Geometry check sheet. Reference: the model listing, model coordinates, mm. A direction names the side the tool comes from. Round coordinates to 2 decimals unless told otherwise and drop trailing zeros. Write each loop counter-clockwise with the first axis right and the second up, starting at its lowest first coordinate (ties: lowest second). Pieces come first, ordered by that corner, then holes. Notation, with made-up numbers: M -36,82 L 9,82 A19 cw 9,118 Z; hole C 51.5,19.5 d5. An arc over 180 degrees is marked long. Answer as CSV lines item,"result". Start each with the question number.
```python
from build123d import *

# Parameters (mm, degrees)
F0_W     = 4.6228
F0_H     = 4.6228
F0_R     = 2.3114
F1_DEPTH = 3.175


with BuildPart() as f1:
    # F0 (on Front) → F1 (new body)
    with BuildSketch(Plane.XZ):
        with BuildLine():
            ThreePointArc((17.3114, -8.3125), (15, -6.0011), (12.6886, -8.3125))
            ThreePointArc((12.6886, -8.3125), (15, -10.6239), (17.3114, -8.3125))
        make_face()
        Polygon((100, -26.9875), (100, 26.9875), (80, 26.9875), (80, 30.1625), (0, 30.1625), (0, -8.3125), (0, -26.9875), align=None)
        with Locations((65.075, -16.3125)):
            Rectangle(F0_W, F0_H, mode=Mode.SUBTRACT)
        with BuildLine():
            ThreePointArc((17.3114, -8.3125), (15, -10.6239), (12.6886, -8.3125))
            ThreePointArc((12.6886, -8.3125), (15, -6.0011), (17.3114, -8.3125))
        make_face(mode=Mode.SUBTRACT)
        with Locations((65.075, -3.6125)):
            Rectangle(F0_W, F0_H, mode=Mode.SUBTRACT)
        with Locations((65.075, 9.0875)):
            Rectangle(F0_W, F0_H, mode=Mode.SUBTRACT)
        Polygon((-65.075, -26.9875), (0, -26.9875), (0, -8.3125), (0, 30.1625), (-80, 30.1625), (-80, 26.9875), (-100, 26.9875), (-100, -26.9875), align=None)
        with Locations((-65.075, -16.3125)):
            Rectangle(F0_W, F0_H, mode=Mode.SUBTRACT)
        with Locations((-65.075, -3.6125)):
            Rectangle(F0_W, F0_H, mode=Mode.SUBTRACT)
        with Locations((-15, -8.3125)):
            Circle(F0_R, mode=Mode.SUBTRACT)
        with Locations((-65.075, 9.0875)):
            Rectangle(F0_W, F0_H, mode=Mode.SUBTRACT)
    extrude(amount=F1_DEPTH)


solid = f1.part
```
1) Section check A-A, the plane x = -15. Record the cut outline in (y, z) (1 decimal), plus the area to 3 significant figures.
2) Scan lines: line 1 (X direction, y = -2.4, z = -4); line 2 (Z direction, x = -15, y = -1.15); line 3 (Z direction, x = 64.5, y = -1.1). Record each from-to range of solid material in increasing order. Write a range as from..to.
3) Section check C-C, the plane y = -1.85. Give the number of separate pieces and of enclosed holes in the cut face, plus the area to 3 significant figures.
4) Access from +Z, -Z, +X, -X, +Y, -Y to the whole of each face (thin tool, end or side, straight path). Record for faces 4 (the flat face through (1, -2, 30.162)), 5 (the flat face through (65, -2, 11.399)).
5) Section check B-B, the plane z = 8.5. Record the cut outline in (x, y) (3 decimals).
6) Mould release check, pull along Z, two halves, no side actions. Record for faces 1 (the flat face through (100, -2, 0)), 2 (the flat face through (-67.386, -2, 9)), 3 (the flat face through (90, -2, 26.988)): released by +Z, released by -Z, zero draft, split by the parting line, or undercut.
Results:
1,outline,"M -3.2,-27 L 0,-27 L 0,-10.6 L -3.2,-10.6 Z; M -3.2,-6 L 0,-6 L 0,30.2 L -3.2,30.2 Z"
1,area,"167 mm^2"
2,line 1,"x = -100..-67.39, -62.76..62.76, 67.39..100"
2,line 2,"z = -26.99..-10.62, -6..30.16"
2,line 3,"z = -26.99..-18.62, -14..-5.92, -1.3..6.78, 11.4..30.16"
3,separate pieces,"1"
3,enclosed holes,"8"
3,area,"11,100 mm^2"
4,face 4,"+Z, +X, -X, +Y, -Y"
4,face 5,"+Y, -Y"
5,outline,"M -100,-3.175 L -67.386,-3.175 L -67.386,0 L -100,0 Z; M -62.764,-3.175 L 62.764,-3.175 L 62.764,0 L -62.764,0 Z; M 67.386,-3.175 L 100,-3.175 L 100,0 L 67.386,0 Z"
6,face 1,"zero draft"
6,face 2,"undercut"
6,face 3,"released by +Z"
